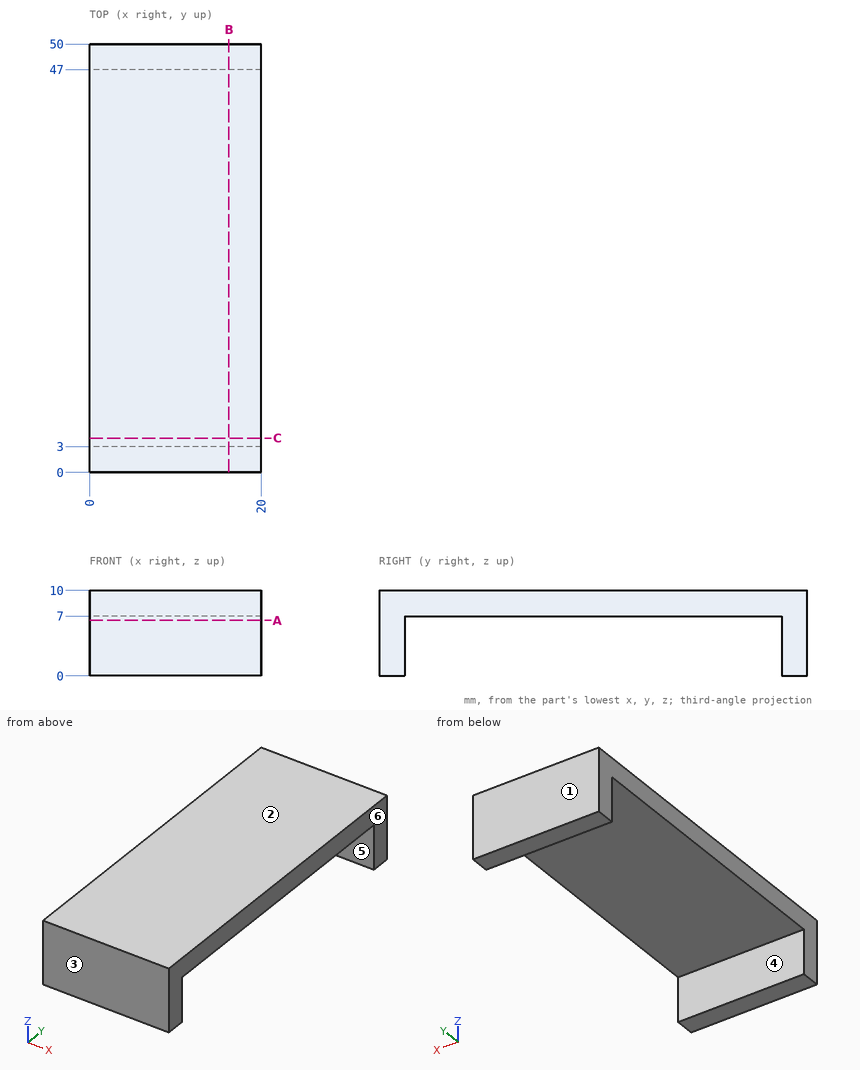
Job drawing, mm, ordinate dimensions from the low corner. One solid piece. A direction names the side the tool comes from. Round coordinates to 2 decimals unless told otherwise and drop trailing zeros. Loops run counter-clockwise (first coordinate to the right, second up) from the corner with the lowest first, then second, coordinate; pieces in that order, holes last.
Item 1: Mould opens along Y. For the marked faces 1, 2, 3 and 4 say: +Y half, -Y half, draft (parallel to the pull), parting line (faces both ways), or undercut.
Item 2: 3-axis set-ups, long thin cutter, end or side, ignore diameter. For the marked faces 5 and 6: which of +Z, -Z, +X, -X, +Y, -Y reach the whole face in a straight line?
Item 3: Cut at A-A, the plane z = 6.5. Give the cut face in (x, y), then the cut area to 3 significant figures.
Item 4: Cut at B-B, the plane x = 16.25. Give the cut face in (y, z).
Item 5: Drill centre lines: line 1 (Y direction, x = 7, z = 6.25); line 2 (Z direction, x = 19, y = 45). Where is each one in solid material? Low to high.
Item 6: Cut at C-C, the plane y = 4. Give the cut face in (x, z).
Item 7: Drop flat-ended pins along their axis: P1, Ø3, axis at x = 17.5, z = 3.5, coming from the -Y side; P2, Ø12, axis at x = 2, y = 37, coming from the -Z side. Give the stop position or say it passes through.
A:
1. face 1: +Y half
1. face 2: draft
1. face 3: -Y half
1. face 4: undercut
2. face 5: -Z, +X, -X
2. face 6: +Z, -Z, +X, +Y, -Y
3. outline: (0, 0) - (20, 0) - (20, 3) - (0, 3) - close; (0, 47) - (20, 47) - (20, 50) - (0, 50) - close
3. area: 120 mm2
4. outline: (0, 0) - (3, 0) - (3, 7) - (47, 7) - (47, 0) - (50, 0) - (50, 10) - (0, 10) - close
5. line 1: y = 0 to 3, 47 to 50
5. line 2: z = 7 to 10
6. outline: (0, 7) - (20, 7) - (20, 10) - (0, 10) - close
7. P1: stops at y = 0
7. P2: stops at z = 7
